```python
from build123d import *

# Parameters (mm, degrees)
F1_DEPTH    = 30
F2_T2_ANGLE = 334.4485965255
F2_T4_ANGLE = 334.4485965255
F4_START    = -10
F4_DEPTH    = 5


# Not quite as in the source:
# - a fillet or chamfer that OpenCascade refuses, or shapes differently, is made with other operations: its cross-section is extruded or revolved along the edge and cut away or added


with BuildPart() as f1:
    # F0 (on Top) → F1 (new body, symmetric)
    with BuildSketch(Plane.XY):
        with BuildLine():
            ThreePointArc((15.0684196329, -7.8703703704), (-17, 0), (15.0684196329, 7.8703703704))
            ThreePointArc((15.0684196329, 7.8703703704), (18.7503186358, 3.9473309343), (23.9321958875, 2.5))
            Line((23.9321958875, 2.5), (36.8151717208, 2.5))
            Line((36.8151717208, 2.5), (36.8151717208, 7.5))
            Line((36.8151717208, 7.5), (23.9321958875, 7.5))
            ThreePointArc((23.9321958875, 7.5), (21.3412572617, 8.2236654671), (19.5003077602, 10.1851851852))
            ThreePointArc((19.5003077602, 10.1851851852), (-22, 0), (19.5003077602, -10.1851851852))
            ThreePointArc((19.5003077602, -10.1851851852), (21.3412572617, -8.2236654671), (23.9321958875, -7.5))
            Line((23.9321958875, -7.5), (36.8151717208, -7.5))
            Line((36.8151717208, -7.5), (36.8151717208, -2.5))
            Line((36.8151717208, -2.5), (23.9321958875, -2.5))
            ThreePointArc((23.9321958875, -2.5), (18.7503186358, -3.9473309343), (15.0684196329, -7.8703703704))
        make_face()
    extrude(amount=F1_DEPTH, both=True)

    # F2: chamfer of 1 on 2 edges, made by hand

    # F2_s1 → F2_t2 (revolve, cut)
    with BuildSketch(Plane(origin=(0, 0, 0), x_dir=(0, 0, 1), z_dir=(0.2211349318, 0.9752432219, 0))):
        Polygon((30, 18), (29, 17), (30, 17), align=None)
    revolve(axis=Axis((0, 0, 30), (0, 0, -1)), revolution_arc=F2_T2_ANGLE, mode=Mode.SUBTRACT)

    # F2_s3 → F2_t4 (revolve, cut)
    with BuildSketch(Plane(origin=(0, 0, 0), x_dir=(0, 0, 1), z_dir=(0.2211349318, 0.9752432219, 0))):
        Polygon((-29, 17), (-30, 18), (-30, 17), align=None)
    revolve(axis=Axis((0, 0, -30), (0, 0, -1)), revolution_arc=F2_T4_ANGLE, mode=Mode.SUBTRACT)

    # F3 (on face) → F4 (join)
    with BuildSketch(Plane(origin=(0, 0, -30), x_dir=(1, 0, 0), z_dir=(0, 0, -1)).offset(F4_START)):
        with BuildLine():
            ThreePointArc((0, -22), (-22, 0), (0, 22))
            Line((0, 22), (-25, 30))
            Line((-25, 30), (-25, -30))
            Line((-25, -30), (0, -22))
        make_face()
    extrude(amount=-F4_DEPTH)

    # F5: F1 across plane


with BuildPart() as f1_1:
    add(f1.part)
    add(f1.part.mirror(Plane.XY))


solid = f1_1.part
```
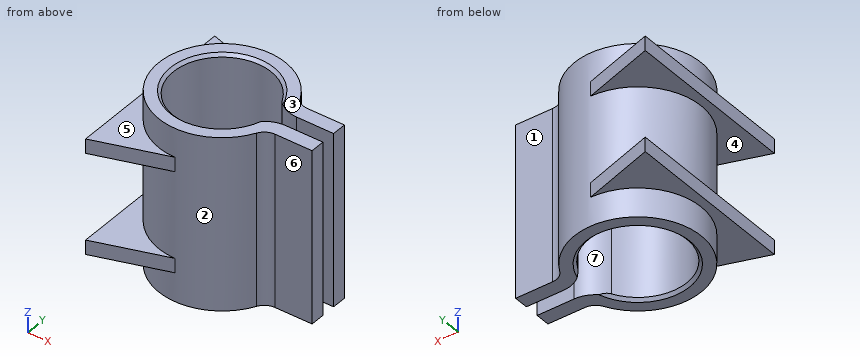
The listing builds one solid part. Answer for the finished solid, in the listing's coordinates (mm). Face numbers are marked on the shaded views. A direction names the side the tool comes from. Coordinates: 2 decimals unless noted, no trailing zeros. Loops run counter-clockwise (first coordinate to the right, second up) from the corner with the lowest first, then second, coordinate; pieces in that order, holes last. Notation, with made-up numbers: (24.25, -32.75) - (65.25, -32.75) arc R13 ccw to (65.25, -16.75) - close; hole circle Ø6 at (55.25, -21). An arc over 180 degrees is marked (long way). Use a Markdown table: item, result. Add a question column.
1) For the marked faces 4, 5, 6 and 7, determine the directions among +Z, -Z, +X, -X, +Y, -Y from which every point of the face is accessible in a straight line to the end or side of a thin tool.
2) Find the intervals of material crossed by line 1 (X direction, y = 0, z = 13.5); line 2 (X direction, y = 9.5, z = -5); line 3 (Y direction, x = 25.5, z = -18), in increasing order.
3) The part is cut by section C-C, the plane y = 0. Give the vertices of the cut face in (x, z), and give its area (3 significant figures).
4) The mould has two halves that part along Z. Classify the marked faces 1, 2 and 3: released by +Z, released by -Z, zero draft, split by the parting line, or undercut.
5) Given pin 1 (10 mm diameter, centred on x = 3.5, y = 9, fed in from +Z); pin 2 (4 mm diameter, centred on x = 30, z = 5.5, fed in from -Y); pin 3 (4 mm diameter, centred on x = 32.5, z = 11.5, fed in from +Y); pin 4 (8 mm diameter, centred on x = 25, z = -1.5, fed in from +Y), each flat-ended and moving along its own axis, determine where each tip first touches the part or whether it passes through.
6) The part is cut by section B-B, the plane z = -0.5. Give the vertices of the cut face in (x, y).
7) The part is cut by section A-A, the plane y = -23. Give the vertices of the cut face in (x, z) (3 decimals), and give its area (3 significant figures).
Here are the results:
| question | item | result |
|---|---|---|
| 1 | face 4 | -X |
| 1 | face 5 | +Z, -X |
| 1 | face 6 | +Z, -Z, +X, -Y |
| 1 | face 7 | +Z, -Z |
| 2 | line 1 | x = -22 to -17 |
| 2 | line 2 | x = -19.84 to -14.1, 14.1 to 19.93 |
| 2 | line 3 | y = -7.5 to -2.5, 2.5 to 7.5 |
| 3 | outline | (-25, -20) - (-22, -20) - (-22, -30) - (-18, -30) - (-17, -29) - (-17, 29) - (-18, 30) - (-22, 30) - (-22, 20) - (-25, 20) - (-25, 15) - (-22, 15) - (-22, -15) - (-25, -15) - close |
| 3 | area | 329 mm^2 |
| 4 | face 1 | zero draft |
| 4 | face 2 | undercut |
| 4 | face 3 | released by +Z |
| 5 | pin 1 | passes through |
| 5 | pin 2 | stops at y = -7.5 |
| 5 | pin 3 | stops at y = 7.5 |
| 5 | pin 4 | stops at y = 8.45 |
| 6 | outline | (15.07, -7.87) arc R17 cw (long way) to (15.07, 7.87) arc R10 ccw to (23.93, 2.5) - (36.82, 2.5) - (36.82, 7.5) - (23.93, 7.5) arc R5 cw to (19.5, 10.19) arc R22 ccw (long way) to (19.5, -10.19) arc R5 cw to (23.93, -7.5) - (36.82, -7.5) - (36.82, -2.5) - (23.93, -2.5) arc R10 ccw to start |
| 7 | outline | (-25, -20) - (-3.125, -20) - (-3.125, -15) - (-25, -15) - close; (-25, 15) - (-3.125, 15) - (-3.125, 20) - (-25, 20) - close |
| 7 | area | 219 mm^2 |
